Geometry check sheet. Reference: the model listing, model coordinates, mm. Face numbers are marked on the shaded views. A direction names the side the tool comes from. Give positions to 0.01 mm unless a question says otherwise; leave off trailing zeros. Order: outer loops, then holes, each group sorted by start corner. A loop starts at its lowest first (then second) coordinate and runs counter-clockwise, first axis right, second up. Notation, with made-up numbers: M -34.75,-12 L -4.75,-12 A36 cw -4.75,22 Z; hole C 71.25,-1 d3. An arc over 180 degrees is marked long. Answer as CSV lines item,"result". Start each with the question number.
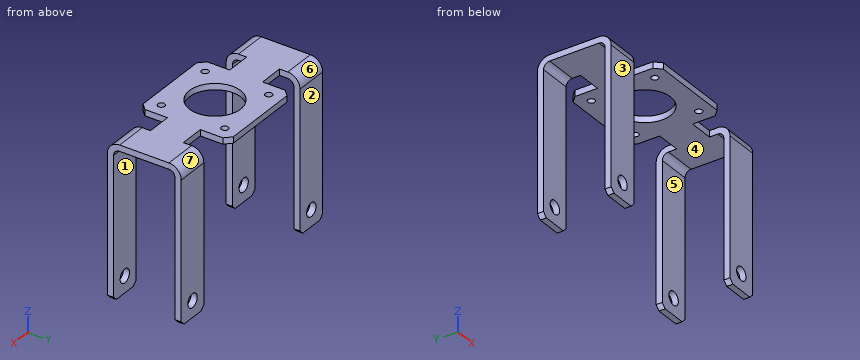
```python
from build123d import *

# Parameters (mm, degrees)
SKETCH_W        = 44
SKETCH_H        = 44
SKETCH_R        = 12.5
SKETCH_R_2      = 1.7
SKETCH_W_2      = 12
SKETCH_H_2      = 16
PAD_DEPTH       = 3
CHAMFER_SIZE    = 3
PAD001_DEPTH    = 16
FILLET_R        = 6
FILLET001_R     = 3
CHAMFER001_SIZE = 2
SKETCH002_R     = 3.3
HOLE_DEPTH      = 40.001


with BuildPart() as part:
    # Sketch → Pad (new body)
    with BuildSketch(Plane.XY):
        Rectangle(SKETCH_W, SKETCH_H)
        Circle(SKETCH_R, mode=Mode.SUBTRACT)
        with Locations((-15.5, 15.5)):
            Circle(SKETCH_R_2, mode=Mode.SUBTRACT)
        with Locations((15.5, 15.5)):
            Circle(SKETCH_R_2, mode=Mode.SUBTRACT)
        with Locations((15.5, -15.5)):
            Circle(SKETCH_R_2, mode=Mode.SUBTRACT)
        with Locations((-15.5, -15.5)):
            Circle(SKETCH_R_2, mode=Mode.SUBTRACT)
        with Locations((28, 0)):
            Rectangle(SKETCH_W_2, SKETCH_H_2)
        with Locations((-28, 0)):
            Rectangle(SKETCH_W_2, SKETCH_H_2)
    extrude(amount=PAD_DEPTH)

    # Chamfer
    chamfer_edges = [part.edges().sort_by_distance(p)[0] for p in [
        (-22, -22, 1.5),
        (22, -22, 1.5),
        (22, 22, 1.5),
        (-22, 22, 1.5),
    ]]
    chamfer(chamfer_edges, length=CHAMFER_SIZE)

    # Sketch001 (on Face11 of Chamfer) → Pad001 (join)
    with BuildSketch(Plane.YZ.offset(34)):
        Polygon((0, 0), (15, 0), (15, -72), (18, -72), (18, 3), (-18, 3), (-18, -72), (-15, -72), (-15, 0), align=None)
    pad001 = extrude(amount=PAD001_DEPTH)

    # Mirrored: Pad001 across YZ
    add(pad001.mirror(Plane.YZ))

    # Fillet
    fillet_edges = [part.edges().sort_by_distance(p)[0] for p in [
        (-42, -18, 3),
        (-42, 18, 3),
        (42, -18, 3),
        (42, 18, 3),
    ]]
    fillet(fillet_edges, radius=FILLET_R)

    # Fillet001
    fillet001_edges = [part.edges().sort_by_distance(p)[0] for p in [
        (-42, 15, 0),
        (42, 15, 0),
        (42, -15, 0),
        (-42, -15, 0),
    ]]
    fillet(fillet001_edges, radius=FILLET001_R)

    # Chamfer001
    chamfer001_edges = [part.edges().sort_by_distance(p)[0] for p in [
        (-50, -16.5, -72),
        (-34, -16.5, -72),
        (-50, 16.5, -72),
        (-34, 16.5, -72),
        (34, -16.5, -72),
        (50, -16.5, -72),
        (34, 16.5, -72),
        (50, 16.5, -72),
    ]]
    chamfer(chamfer001_edges, length=CHAMFER001_SIZE)

    # Sketch002 (on Face46 of Chamfer001) → Hole (cut, through all)
    with BuildSketch(Plane.XZ.offset(18)):
        with Locations((-42, -64)):
            Circle(SKETCH002_R)
        with Locations((42, -64)):
            Circle(SKETCH002_R)
    extrude(amount=-HOLE_DEPTH, mode=Mode.SUBTRACT)


solid = part.part
```
Item 1: Draft check along Y on the marked faces 1, 2 and 3. Enter one of: pulls with the +Y half, pulls with the -Y half, needs draft (parallel to the pull), parting line crosses it, or undercut.
Item 2: Section check A-A on x = -42. Record the boundary of the cut face in (y, z), then the cut area to 3 significant figures.
Item 3: Scan lines: line 1 along Y through (x, z) = (15.5, 0.75); line 2 along X through (y, z) = (-15.5, -45.5); line 3 along Y through (x, z) = (35, -31). Record each from-to range of solid material in increasing order.
Item 4: Section check D-D on x = 3.5. Record the boundary of the cut face in (y, z), then the cut area to 3 significant figures.
Item 5: Depth check by flat-ended pin: pin 1 Ø0.9 at (x, z) = (30.5, 1) entering from -Y; pin 2 Ø5 at (x, z) = (45, -23.5) entering from +Y; pin 3 Ø13 at (x, z) = (-41.5, -40) entering from -Y. Enter the tip coordinate at first touch or a pass-through.
Item 6: Section check B-B on y = -10. Record the boundary of the cut face in (x, z), then the cut area to 3 significant figures.
Item 7: Section check C-C on z = -21. Record the boundary of the cut face in (x, y).
Item 8: Access from +Z, -Z, +X, -X, +Y, -Y to the whole of each face (thin tool, end or side, straight path). Record for the marked faces 4, 5, 6 and 7.
Numbers:
1,face 1,"undercut"
1,face 2,"pulls with the +Y half"
1,face 3,"pulls with the -Y half"
2,outline,"M -18,-72 L -15,-72 L -15,-67.3 L -18,-67.3 Z; M -18,-60.7 L -15,-60.7 L -15,-3 A3 cw -12,0 L 12,0 A3 cw 15,-3 L 15,-60.7 L 18,-60.7 L 18,-3 A6 ccw 12,3 L -12,3 A6 ccw -18,-3 Z; M 15,-72 L 18,-72 L 18,-67.3 L 15,-67.3 Z"
2,area,"489 mm2"
3,line 1,"-22 to -17.2, -13.8 to 13.8, 17.2 to 22"
3,line 2,"-50 to -34, 34 to 50"
3,line 3,"-18 to -15, 15 to 18"
4,outline,"M -22,0 L -12,0 L -12,3 L -22,3 Z; M 12,0 L 22,0 L 22,3 L 12,3 Z"
4,area,"60.0 mm2"
5,pin 1,"y = -8"
5,pin 2,"y = 18"
5,pin 3,"y = -18"
6,outline,"M -50,0 L -34,0 L -34,3 L -50,3 Z; M -22,0 L -7.5,0 L -7.5,3 L -22,3 Z; M 7.5,0 L 22,0 L 22,3 L 7.5,3 Z; M 34,0 L 50,0 L 50,3 L 34,3 Z"
6,area,"183 mm2"
7,outline,"M -50,-18 L -34,-18 L -34,-15 L -50,-15 Z; M -50,15 L -34,15 L -34,18 L -50,18 Z; M 34,-18 L 50,-18 L 50,-15 L 34,-15 Z; M 34,15 L 50,15 L 50,18 L 34,18 Z"
8,face 4,"-Z"
8,face 5,"-Z, +X, -X"
8,face 6,"+Z, -X, +Y"
8,face 7,"+Z, +X, +Y"
